Input: part model. Units: mm. Frame: model coordinates. A direction names the side the tool comes from. Coordinates: 2 decimals unless noted, no trailing zeros. Loops run counter-clockwise (first coordinate to the right, second up) from the corner with the lowest first, then second, coordinate; pieces in that order, holes last.
(1) Section B-B, the plane y = 0. Return loops of the section in (x, z), then the cut area to 3 significant figures.
(2) Section D-D, the plane x = -28. Return loops of the section in (y, z).
(3) Mould query, pull axis X, two halves, no side actions, for faces 1 (the face through (41, -3, 1)), 2 (the face through (-37, -14, 1)), 3 (the face through (-30, -14, 1)). Classes: released by +X, released by -X, zero draft, split by the parting line, or undercut.
(4) Line query: L1, parallel to Y at x = 0, z = 0.95; L2, parallel to Y at x = -7.5, z = 1.45; L3, parallel to Y at x = 33.5, z = 0.25. Output: solid intervals per line, ascending.
(5) Contact query for flat-ended pins moving along their axis: P1, Ø5, axis at x = -7.5, y = 12.99, coming from the +Z side; P2, Ø1, axis at x = -28, z = 0.5, coming from the -Y side; P3, Ø0.6, axis at x = 35, z = 1, coming from the -Y side; P4, Ø2, axis at x = -23.5, y = -16.5, coming from the +Z side. Output: stop coordinate, or through.
(6) Set-up query: faces 4 (the face through (40, 1.5, 1)), 5 (the face through (-41, -11, 1)), 6 (the face through (39, -12.75, 1)). Return all of +Z, -Z, +X, -X, +Y, -Y with unobstructed straight access to the full face (end or side cutting, diameter ignored); none if empty.
(7) Section A-A, the plane x = -4. Return loops of the section in (y, z).
(8) Section C-C, the plane x = 7.5. Return loops of the section in (y, z), then the cut area to 3 significant figures.
```python
from build123d import *

# Parameters (mm, degrees)
SKETCH_1_R      = 2
SKETCH_1_R_2    = 2.08
SKETCH_1_R_3    = 8.75
EXTRUDE_2_DEPTH = 2


with BuildPart() as part:
    # 草图1 → 凸台-拉伸2 (new body)
    with BuildSketch(Plane.XY):
        with BuildLine():
            Line((-30, 12.75), (-25.488968202, 12.75))
            ThreePointArc((-25.488968202, 12.75), (0, 23.30787632), (25.488968202, 12.75))
            Line((25.488968202, 12.75), (30, 12.75))
            Line((30, 12.75), (30, 15.75))
            Line((30, 15.75), (37, 15.75))
            Line((37, 15.75), (37, 12.75))
            Line((37, 12.75), (41, 12.75))
            Line((41, 12.75), (41, 9.5))
            Line((41, 9.5), (44, 9.5))
            Line((44, 9.5), (44, 4.5))
            Line((44, 4.5), (41, 4.5))
            Line((41, 4.5), (41, 1.5))
            Line((41, 1.5), (38.5, 1.5))
            Line((38.5, 1.5), (38.5, 3))
            Line((38.5, 3), (35.9, 3))
            Line((35.9, 3), (35.9, 1.5))
            Line((35.9, 1.5), (32.9, 1.5))
            Line((32.9, 1.5), (32.9, -1.5))
            Line((32.9, -1.5), (35.9, -1.5))
            Line((35.9, -1.5), (35.9, -3))
            Line((35.9, -3), (38.5, -3))
            Line((38.5, -3), (38.5, -1.5))
            Line((38.5, -1.5), (41, -1.5))
            Line((41, -1.5), (41, -4.5))
            Line((41, -4.5), (44, -4.5))
            Line((44, -4.5), (44, -9.5))
            Line((44, -9.5), (41, -9.5))
            Line((41, -9.5), (41, -11.75))
            Line((41, -11.75), (40, -12.75))
            Line((40, -12.75), (37, -12.75))
            Line((37, -12.75), (37, -15.75))
            Line((37, -15.75), (30, -15.75))
            Line((30, -15.75), (30, -12.75))
            Line((30, -12.75), (25.488968202, -12.75))
            ThreePointArc((25.488968202, -12.75), (0, -23.30787632), (-25.488968202, -12.75))
            Line((-25.488968202, -12.75), (-30, -12.75))
            Line((-30, -12.75), (-30, -15.75))
            Line((-30, -15.75), (-37, -15.75))
            Line((-37, -15.75), (-37, -12.75))
            Line((-37, -12.75), (-41, -12.75))
            Line((-41, -12.75), (-41, -9.5))
            Line((-41, -9.5), (-44, -9.5))
            Line((-44, -9.5), (-44, -4.5))
            Line((-44, -4.5), (-41, -4.5))
            Line((-41, -4.5), (-41, -1.5))
            Line((-41, -1.5), (-38.5, -1.5))
            Line((-38.5, -1.5), (-38.5, -3))
            Line((-38.5, -3), (-35.9, -3))
            Line((-35.9, -3), (-35.9, -1.5))
            Line((-35.9, -1.5), (-32.9, -1.5))
            Line((-32.9, -1.5), (-32.9, 1.5))
            Line((-32.9, 1.5), (-35.9, 1.5))
            Line((-35.9, 1.5), (-35.9, 3))
            Line((-35.9, 3), (-38.5, 3))
            Line((-38.5, 3), (-38.5, 1.5))
            Line((-38.5, 1.5), (-41, 1.5))
            Line((-41, 1.5), (-41, 4.5))
            Line((-41, 4.5), (-44, 4.5))
            Line((-44, 4.5), (-44, 9.5))
            Line((-44, 9.5), (-41, 9.5))
            Line((-41, 9.5), (-41, 12.75))
            Line((-41, 12.75), (-37, 12.75))
            Line((-37, 12.75), (-37, 15.75))
            Line((-37, 15.75), (-30, 15.75))
            Line((-30, 15.75), (-30, 12.75))
        make_face()
        with Locations((-15, 0)):
            Circle(SKETCH_1_R, mode=Mode.SUBTRACT)
        with Locations((-7.5, 12.990381057)):
            Circle(SKETCH_1_R, mode=Mode.SUBTRACT)
        with Locations((7.5, 12.990381057)):
            Circle(SKETCH_1_R, mode=Mode.SUBTRACT)
        with Locations((15, 0)):
            Circle(SKETCH_1_R, mode=Mode.SUBTRACT)
        with Locations((7.5, -12.990381057)):
            Circle(SKETCH_1_R, mode=Mode.SUBTRACT)
        with Locations((-7.5, -12.990381057)):
            Circle(SKETCH_1_R, mode=Mode.SUBTRACT)
        with Locations((0, 13.53)):
            Circle(SKETCH_1_R_2, mode=Mode.SUBTRACT)
        with Locations((11.717323713, -6.765)):
            Circle(SKETCH_1_R_2, mode=Mode.SUBTRACT)
        with Locations((-11.717323713, -6.765)):
            Circle(SKETCH_1_R_2, mode=Mode.SUBTRACT)
        Circle(SKETCH_1_R_3, mode=Mode.SUBTRACT)
    extrude(amount=EXTRUDE_2_DEPTH)


solid = part.part
```
Report:
1. outline: (-32.9, 0) - (-17, 0) - (-17, 2) - (-32.9, 2) - close; (-13, 0) - (-8.75, 0) - (-8.75, 2) - (-13, 2) - close; (8.75, 0) - (13, 0) - (13, 2) - (8.75, 2) - close; (17, 0) - (32.9, 0) - (32.9, 2) - (17, 2) - close
1. area: 80.6 mm2
2. outline: (-12.75, 0) - (12.75, 0) - (12.75, 2) - (-12.75, 2) - close
3. face 1: released by +X
3. face 2: released by -X
3. face 3: undercut
4. L1: y = -23.31 to -8.75, 8.75 to 11.45, 15.61 to 23.31
4. L2: y = -22.52 to -14.99, -10.99 to -4.51, 4.51 to 10.99, 14.99 to 22.52
4. L3: y = -15.75 to -1.5, 1.5 to 15.75
5. P1: stops at z = 2
5. P2: stops at y = -12.75
5. P3: stops at y = -15.75
5. P4: passes through
6. face 4: +Z, -Z, +X
6. face 5: +Z, -Z, -X, -Y
6. face 6: +Z, -Z, +X, -Y
7. outline: (-23.09, 0) - (-7.78, 0) - (-7.78, 2) - (-23.09, 2) - close; (7.78, 0) - (23.09, 0) - (23.09, 2) - (7.78, 2) - close
8. outline: (-22.52, 0) - (-14.99, 0) - (-14.99, 2) - (-22.52, 2) - close; (-10.99, 0) - (-4.51, 0) - (-4.51, 2) - (-10.99, 2) - close; (4.51, 0) - (10.99, 0) - (10.99, 2) - (4.51, 2) - close; (14.99, 0) - (22.52, 0) - (22.52, 2) - (14.99, 2) - close
8. area: 56.0 mm2
